```python
from build123d import *

# Parameters (mm, degrees)
F1_DEPTH = 0.2


with BuildPart() as f1:
    # F0 (on Top) → F1 (new body)
    with BuildSketch(Plane.XY):
        Polygon((-0.15, -0.0621320344), (-0.0621320344, -0.15), (0, -0.15), (0.0621320344, -0.15), (0.15, -0.0621320344), (0.15, 0), (0.15, 0.0621320344), (0.0621320344, 0.15), (0, 0.15), (-0.0621320344, 0.15), (-0.15, 0.0621320344), (-0.15, 0), align=None)
        Polygon((0, 0.2121320344), (-0.0621320344, 0.15), (0, 0.15), (0.0621320344, 0.15), align=None)
        Polygon((0.15, 0), (0.15, -0.0621320344), (0.2121320344, 0), (0.15, 0.0621320344), align=None)
        Polygon((0.0621320344, -0.15), (0.15, -0.15), (0.15, -0.0621320344), align=None)
        Polygon((0.0621320344, 0.15), (0.15, 0.0621320344), (0.15, 0.15), align=None)
        Polygon((0.15, 0.0621320344), (0.2121320344, 0), (0.3621320344, 0.15), (0.15, 0.15), align=None)
        Polygon((0, 0.2121320344), (0.0621320344, 0.15), (0.15, 0.15), (0.15, 0.3621320344), align=None)
        Polygon((0.15, -0.0621320344), (0.15, -0.15), (0.3621320344, -0.15), (0.2121320344, 0), align=None)
        with BuildLine():
            Line((0.3621320344, -0.15), (22.3494966386, -0.15))
            ThreePointArc((22.3494966386, -0.15), (22.3498741593, -0.0750004223), (22.35, 0))
            ThreePointArc((22.35, 0), (22.3498741593, 0.0750004223), (22.3494966386, 0.15))
            Line((22.3494966386, 0.15), (0.3621320344, 0.15))
            Line((0.3621320344, 0.15), (0.2121320344, 0))
            Line((0.2121320344, 0), (0.3621320344, -0.15))
        make_face()
        with BuildLine():
            Line((0.15, 0.15), (0.3621320344, 0.15))
            Line((0.3621320344, 0.15), (15.9095466465, 15.6974146121))
            ThreePointArc((15.9095466465, 15.6974146121), (15.8038365595, 15.8038365595), (15.6974146121, 15.9095466465))
            Line((15.6974146121, 15.9095466465), (0.15, 0.3621320344))
            Line((0.15, 0.3621320344), (0.15, 0.15))
        make_face()
        with BuildLine():
            ThreePointArc((0.15, 22.3494966386), (0, 22.35), (-0.15, 22.3494966386))
            Line((-0.15, 22.3494966386), (-0.15, 0.3621320344))
            Line((-0.15, 0.3621320344), (0, 0.2121320344))
            Line((0, 0.2121320344), (0.15, 0.3621320344))
            Line((0.15, 0.3621320344), (0.15, 22.3494966386))
        make_face()
        Polygon((0, -0.2121320344), (0.15, -0.3621320344), (0.15, -0.15), (0.0621320344, -0.15), align=None)
        with BuildLine():
            Line((0.15, -0.3621320344), (15.6974146121, -15.9095466465))
            ThreePointArc((15.6974146121, -15.9095466465), (15.8038365595, -15.8038365595), (15.9095466465, -15.6974146121))
            Line((15.9095466465, -15.6974146121), (0.3621320344, -0.15))
            Line((0.3621320344, -0.15), (0.15, -0.15))
            Line((0.15, -0.15), (0.15, -0.3621320344))
        make_face()
        Polygon((-0.0621320344, -0.15), (0, -0.2121320344), (0.0621320344, -0.15), (0, -0.15), align=None)
        Polygon((-0.15, -0.15), (-0.15, -0.3621320344), (0, -0.2121320344), (-0.0621320344, -0.15), align=None)
        Polygon((-0.15, -0.0621320344), (-0.15, -0.15), (-0.0621320344, -0.15), align=None)
        Polygon((-0.2121320344, 0), (-0.15, -0.0621320344), (-0.15, 0), (-0.15, 0.0621320344), align=None)
        Polygon((-0.15, 0.3621320344), (-0.15, 0.15), (-0.0621320344, 0.15), (0, 0.2121320344), align=None)
        Polygon((-0.15, 0.15), (-0.15, 0.0621320344), (-0.0621320344, 0.15), align=None)
        Polygon((-0.3621320344, 0.15), (-0.2121320344, 0), (-0.15, 0.0621320344), (-0.15, 0.15), align=None)
        with BuildLine():
            ThreePointArc((-15.6974146121, 15.9095466465), (-15.8038365595, 15.8038365595), (-15.9095466465, 15.6974146121))
            Line((-15.9095466465, 15.6974146121), (-0.3621320344, 0.15))
            Line((-0.3621320344, 0.15), (-0.15, 0.15))
            Line((-0.15, 0.15), (-0.15, 0.3621320344))
            Line((-0.15, 0.3621320344), (-15.6974146121, 15.9095466465))
        make_face()
        with BuildLine():
            ThreePointArc((-22.3494966386, 0.15), (-22.35, 0), (-22.3494966386, -0.15))
            Line((-22.3494966386, -0.15), (-0.3621320344, -0.15))
            Line((-0.3621320344, -0.15), (-0.2121320344, 0))
            Line((-0.2121320344, 0), (-0.3621320344, 0.15))
            Line((-0.3621320344, 0.15), (-22.3494966386, 0.15))
        make_face()
        Polygon((-0.3621320344, -0.15), (-0.15, -0.15), (-0.15, -0.0621320344), (-0.2121320344, 0), align=None)
        with BuildLine():
            ThreePointArc((-15.9095466465, -15.6974146121), (-15.8038365595, -15.8038365595), (-15.6974146121, -15.9095466465))
            Line((-15.6974146121, -15.9095466465), (-0.15, -0.3621320344))
            Line((-0.15, -0.3621320344), (-0.15, -0.15))
            Line((-0.15, -0.15), (-0.3621320344, -0.15))
            Line((-0.3621320344, -0.15), (-15.9095466465, -15.6974146121))
        make_face()
        with BuildLine():
            Line((-0.15, -0.3621320344), (-0.15, -22.3494966386))
            ThreePointArc((-0.15, -22.3494966386), (0, -22.35), (0.15, -22.3494966386))
            Line((0.15, -22.3494966386), (0.15, -0.3621320344))
            Line((0.15, -0.3621320344), (0, -0.2121320344))
            Line((0, -0.2121320344), (-0.15, -0.3621320344))
        make_face()
        with BuildLine():
            Line((-0.15, -22.3494966386), (-0.15, -22.4994999944))
            ThreePointArc((-0.15, -22.4994999944), (0, -22.5), (0.15, -22.4994999944))
            Line((0.15, -22.4994999944), (0.15, -22.3494966386))
            ThreePointArc((0.15, -22.3494966386), (0, -22.35), (-0.15, -22.3494966386))
        make_face()
        with BuildLine():
            ThreePointArc((0.15, -22.4994999944), (15.9628474903, -15.8567808839), (22.5, 0))
            ThreePointArc((22.5, 0), (-15.8567808839, 15.9628474903), (-0.15, -22.4994999944))
            Line((-0.15, -22.4994999944), (-0.15, -22.3494966386))
            ThreePointArc((-0.15, -22.3494966386), (-8.5529747134, -20.6487075516), (-15.6974146121, -15.9095466465))
            ThreePointArc((-15.6974146121, -15.9095466465), (-15.8038365595, -15.8038365595), (-15.9095466465, -15.6974146121))
            ThreePointArc((-15.9095466465, -15.6974146121), (-20.6487075516, -8.5529747134), (-22.3494966386, -0.15))
            ThreePointArc((-22.3494966386, -0.15), (-22.35, 0), (-22.3494966386, 0.15))
            ThreePointArc((-22.3494966386, 0.15), (-20.6487075516, 8.5529747134), (-15.9095466465, 15.6974146121))
            ThreePointArc((-15.9095466465, 15.6974146121), (-15.8038365595, 15.8038365595), (-15.6974146121, 15.9095466465))
            ThreePointArc((-15.6974146121, 15.9095466465), (-8.5529747134, 20.6487075516), (-0.15, 22.3494966386))
            ThreePointArc((-0.15, 22.3494966386), (0, 22.35), (0.15, 22.3494966386))
            ThreePointArc((0.15, 22.3494966386), (8.5529747134, 20.6487075516), (15.6974146121, 15.9095466465))
            ThreePointArc((15.6974146121, 15.9095466465), (15.8038365595, 15.8038365595), (15.9095466465, 15.6974146121))
            ThreePointArc((15.9095466465, 15.6974146121), (20.6487075516, 8.5529747134), (22.3494966386, 0.15))
            ThreePointArc((22.3494966386, 0.15), (22.3498741593, 0.0750004223), (22.35, 0))
            ThreePointArc((22.35, 0), (22.3498741593, -0.0750004223), (22.3494966386, -0.15))
            ThreePointArc((22.3494966386, -0.15), (20.6487075516, -8.5529747134), (15.9095466465, -15.6974146121))
            ThreePointArc((15.9095466465, -15.6974146121), (15.8038365595, -15.8038365595), (15.6974146121, -15.9095466465))
            ThreePointArc((15.6974146121, -15.9095466465), (8.5529747134, -20.6487075516), (0.15, -22.3494966386))
            Line((0.15, -22.3494966386), (0.15, -22.4994999944))
        make_face()
    extrude(amount=F1_DEPTH)


solid = f1.part
```
Input: part model. Units: mm. Frame: model coordinates. Round coordinates to 2 decimals unless told otherwise and drop trailing zeros. Order: outer loops, then holes, each group sorted by start corner. A loop starts at its lowest first (then second) coordinate and runs counter-clockwise, first axis right, second up. Notation, with made-up numbers: (-30, -27) - (6, -27) arc R12 ccw to (6, -8) - close; hole circle Ø7 at (6.5, -1). An arc over 180 degrees is marked (long way). One line per question, with ' | ' between items. Start each with the question number.
1) Contact query for a flat-ended pin moving along its axis: P1, Ø1, axis at x = 11, y = -2, coming from the -Z side. Output: stop coordinate, or through.
2) Cut plane A-A, the plane z = 0.1. Give the number of separate pieces and of enclosed holes in the cut face, then the cut area to 3 significant figures.
3) Cut plane C-C, the plane y = 18.5. Return the cut outline in (x, z), then the cut area to 3 significant figures.
4) Cut plane D-D, the plane y = 5.5. Return the cut outline in (x, z).
5) Ray query, probe 1 along X at (y, z) = (-3.5, 0.1); probe 2 along X at (y, z) = (16.5, 0.1); probe 3 along X at (y, z) = (4.5, 0.1). Return the intervals inside material, ascending.
6) Cut plane B-B, the plane x = -19. Return the cut outline in (y, z).
Worked out:
1) P1: passes through
2) separate pieces: 1 | enclosed holes: 8 | area: 74.3 mm^2
3) outline: (-12.81, 0) - (-12.54, 0) - (-12.54, 0.2) - (-12.81, 0.2) - close; (-0.15, 0) - (0.15, 0) - (0.15, 0.2) - (-0.15, 0.2) - close; (12.54, 0) - (12.81, 0) - (12.81, 0.2) - (12.54, 0.2) - close | area: 0.166 mm^2
4) outline: (-21.82, 0) - (-21.66, 0) - (-21.66, 0.2) - (-21.82, 0.2) - close; (-5.71, 0) - (-5.29, 0) - (-5.29, 0.2) - (-5.71, 0.2) - close; (-0.15, 0) - (0.15, 0) - (0.15, 0.2) - (-0.15, 0.2) - close; (5.29, 0) - (5.71, 0) - (5.71, 0.2) - (5.29, 0.2) - close; (21.66, 0) - (21.82, 0) - (21.82, 0.2) - (21.66, 0.2) - close
5) probe 1: x = -22.23 to -22.07, -3.71 to -3.29, -0.15 to 0.15, 3.29 to 3.71, 22.07 to 22.23 | probe 2: x = -15.3 to -15.08, -0.15 to 0.15, 15.08 to 15.3 | probe 3: x = -22.05 to -21.89, -4.71 to -4.29, -0.15 to 0.15, 4.29 to 4.71, 21.89 to 22.05
6) outline: (-12.05, 0) - (-11.77, 0) - (-11.77, 0.2) - (-12.05, 0.2) - close; (-0.15, 0) - (0.15, 0) - (0.15, 0.2) - (-0.15, 0.2) - close; (11.77, 0) - (12.05, 0) - (12.05, 0.2) - (11.77, 0.2) - close
